from build123d import *

# Parameters (mm, degrees)
F1_DEPTH      = 15.08125
F1_DEPTH_BACK = 15.08125
F2_R          = 63.5
F3_R          = 22.225
F4_R          = 12.7


with BuildPart() as f1:
    # F0 (on Right) → F1 (new body, two sides)
    with BuildSketch(Plane.YZ) as f1_sk:
        Polygon((0, 14.2875), (0, 0), (271.4625, 0), (271.4625, 30.48), (390.525, 30.48), (390.525, 0), (488.95, 0), (488.95, 30.48), (608.0125, 30.48), (608.0125, 0), (711.2, 0), (711.2, 30.48), (830.2625, 30.48), (830.2625, 0), (892.175, 0), (892.175, 38.1), (866.775, 51.60542), (830.2625, 63.5), (271.4625, 63.5), (25.4, 25.06916), align=None)
    extrude(amount=F1_DEPTH)
    extrude(f1_sk.sketch, amount=-F1_DEPTH_BACK)

    # F2
    f2_edges = [f1.edges().sort_by_distance(p)[0] for p in [
        (0, 25.4, 25.06916),
        (0, 271.4625, 63.5),
        (0, 830.2625, 63.5),
        (0, 866.775, 51.60542),
    ]]
    fillet(f2_edges, radius=F2_R)

    # F3
    f3_edges = [f1.edges().sort_by_distance(p)[0] for p in [
        (0, 271.4625, 30.48),
        (0, 488.95, 30.48),
        (0, 711.2, 30.48),
        (0, 390.525, 30.48),
        (0, 608.0125, 30.48),
        (0, 830.2625, 30.48),
    ]]
    fillet(f3_edges, radius=F3_R)

    # F4
    f4_edges = [f1.edges().sort_by_distance(p)[0] for p in [
        (-15.08125, 330.99375, 30.48),
        (15.08125, 330.99375, 30.48),
        (-15.08125, 548.48125, 30.48),
        (15.08125, 548.48125, 30.48),
        (-15.08125, 770.73125, 30.48),
        (15.08125, 770.73125, 30.48),
        (15.08125, 548.28579, 63.5),
        (-15.08125, 548.28579, 63.5),
    ]]
    fillet(f4_edges, radius=F4_R)


solid = f1.part
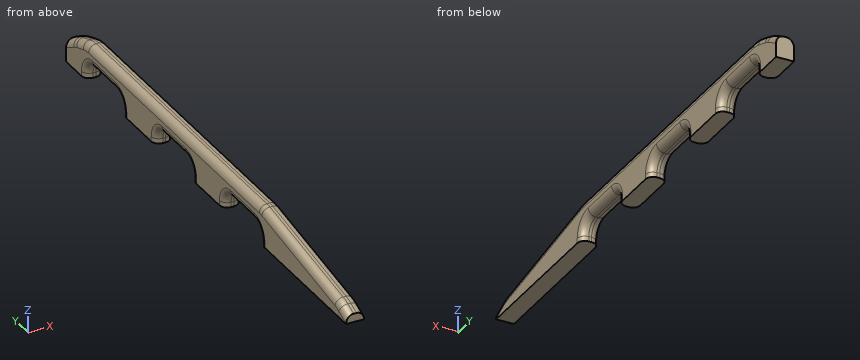
Verification items for the finished model (mm, model axes). Give positions to 0.01 mm unless a question says otherwise; leave off trailing zeros. Write each loop counter-clockwise with the first axis right and the second up, starting at its lowest first coordinate (ties: lowest second). Pieces come first, ordered by that corner, then holes.
(1) Cross-section at A-A (y = 314). Enter the section's corners in (x, z), plus the area to 3 significant figures.
(2) Material ranges on line 1 (Y direction, x = 1.5, z = 17) (3 decimals); line 2 (Y direction, x = -7, z = 8) (3 decimals); line 3 (Z direction, x = 11, y = 202), recorded low to high.
(3) Gauge pin test, flat ends, axial feed: pin 1 (2.5 mm diameter, centred on x = 0.5, y = 769.5, fed in from -Z); pin 2 (10 mm diameter, centred on x = 0, z = 24.5, fed in from -Y); pin 3 (12 mm diameter, centred on y = 544, z = 35.5, fed in from -X). Record the tip position at first contact, or that the pin passes through.
Worked out:
1. outline: (-15.08, 43.18) arc R12.7 ccw to (-2.38, 30.48) - (2.38, 30.48) arc R12.7 ccw to (15.08, 43.18) - (15.08, 50.8) arc R12.7 ccw to (2.38, 63.5) - (-2.38, 63.5) arc R12.7 ccw to (-15.08, 50.8) - close
1. area: 858 mm2
2. line 1: y = 6.39 to 273.255, 388.732 to 490.743, 606.22 to 712.993, 828.47 to 892.175
2. line 2: y = 0 to 270.593, 391.395 to 488.08, 608.882 to 710.33, 831.132 to 892.175
2. line 3: z = 0 to 49.24
3. pin 1: stops at z = 30.48
3. pin 2: stops at y = 12.28
3. pin 3: stops at x = -14.97
